Verification items for this drawing (mm, ordinates from the low corner). Give positions to 0.01 mm unless a question says otherwise; leave off trailing zeros. Loops run counter-clockwise (first coordinate to the right, second up) from the corner with the lowest first, then second, coordinate; pieces in that order, holes last. Notation, with made-up numbers: (58.25, -31.75) -> (106.25, -31.75) arc R27 ccw to (106.25, 3.25) -> close; hole circle Ø10 at (20.5, 30). An arc over 180 degrees is marked (long way). Write each question's results on one line, items separated by ' | '. Start each with the question number.
Item 1: Scan lines: line 1 along Y through (x, z) = (187.5, 0.85); line 2 along X through (y, z) = (82, 1). Record each from-to range of solid material in increasing order.
Item 2: Cross-section at A-A on y = 118. Enter the section's corners in (x, z), then the cut area to 3 significant figures.
Item 3: Gauge pin test, flat ends, axial feed: pin 1 Ø0.9 at (x, z) = (248.5, 1.5) entering from +Y; pin 2 Ø1.5 at (y, z) = (158, 1) entering from +X; pin 3 Ø0.9 at (y, z) = (1, 2) entering from -X. Record the tip position at first contact, or that the pin passes through.
Item 4: Cross-section at B-B on x = 180.5. Enter the section's corners in (y, z), then the cut area to 3 significant figures.
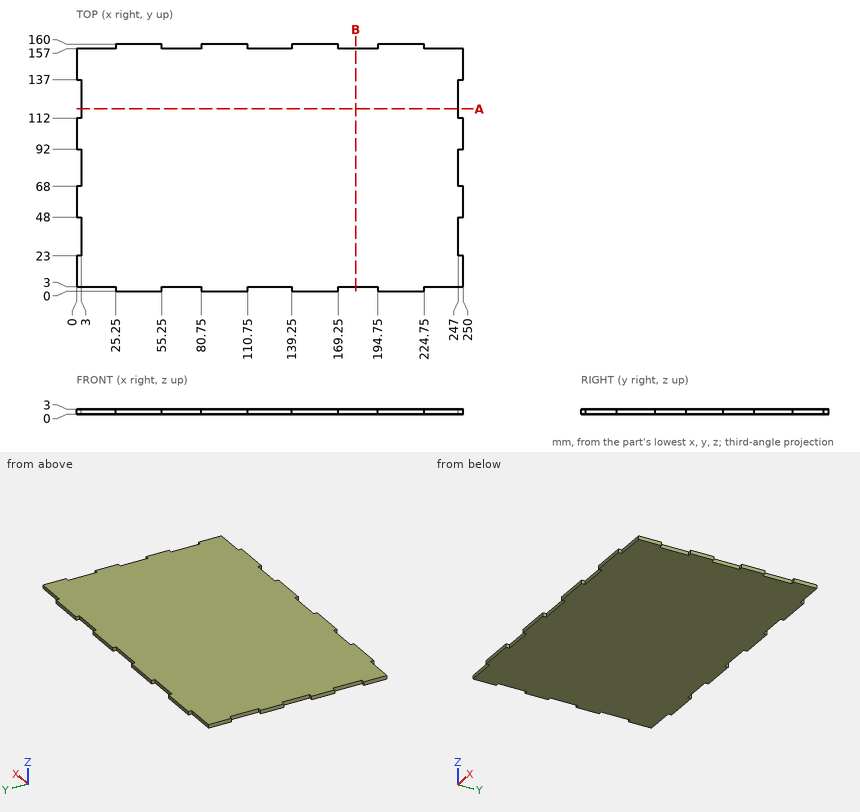
Answer sheet:
1) line 1: y = 3 to 157 | line 2: x = 3 to 247
2) outline: (3, 0) -> (247, 0) -> (247, 3) -> (3, 3) -> close | area: 732 mm²
3) pin 1: stops at y = 157 | pin 2: stops at x = 224.75 | pin 3: stops at x = 25.25
4) outline: (3, 0) -> (157, 0) -> (157, 3) -> (3, 3) -> close | area: 462 mm²
